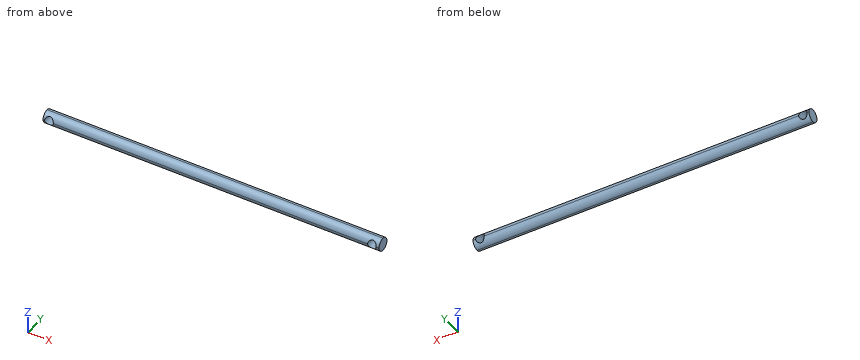
from build123d import *

# Parameters (mm, degrees)
F0_W        = 390
F0_H        = 15
F1_DEPTH    = 15
F2_R        = 5
F3_DEPTH    = 20
F4_T1_DEPTH = 430


# Not quite as in the source:
# - a fillet or chamfer that OpenCascade refuses, or shapes differently, is made with other operations: its cross-section is extruded or revolved along the edge and cut away or added


with BuildPart() as f1:
    # F0 (on Front) → F1 (new body)
    with BuildSketch(Plane.XZ):
        with Locations((-195, 7.5)):
            Rectangle(F0_W, F0_H)
    extrude(amount=F1_DEPTH)

    # F2 (on Front) → F3 (cut)
    with BuildSketch(Plane.XZ):
        with Locations((-383.0693596974, 7.6079843566)):
            Circle(F2_R)
        with Locations((-8.0693596974, 7.6553751715)):
            Circle(F2_R)
    extrude(amount=F3_DEPTH, mode=Mode.SUBTRACT)

    # F4: fillet of radius 8 on 4 edges, made by hand

    # F4_s2 → F4_t1 (cut)
    with BuildSketch(Plane.YZ.offset(-410)):
        with BuildLine():
            ThreePointArc((-8, 15), (-2.3431457505, 12.6568542495), (0, 7))
            Line((0, 7), (0, 15))
            Line((0, 15), (-8, 15))
        make_face()
        with BuildLine():
            ThreePointArc((0, 8), (-2.3431457505, 2.3431457505), (-8, 0))
            Line((-8, 0), (0, 0))
            Line((0, 0), (0, 8))
        make_face()
        with BuildLine():
            ThreePointArc((-7, 15), (-12.6568542495, 12.6568542495), (-15, 7))
            Line((-15, 7), (-15, 15))
            Line((-15, 15), (-7, 15))
        make_face()
        with BuildLine():
            ThreePointArc((-15, 8), (-12.6568542495, 2.3431457505), (-7, 0))
            Line((-7, 0), (-15, 0))
            Line((-15, 0), (-15, 8))
        make_face()
    extrude(amount=F4_T1_DEPTH, mode=Mode.SUBTRACT)


solid = f1.part
Check sheet for the modelled part. Datum: model origin and axes. Units: mm. Round coordinates to 2 decimals unless told otherwise and drop trailing zeros. Loops run counter-clockwise (first coordinate to the right, second up) from the corner with the lowest first, then second, coordinate; pieces in that order, holes last. Notation, with made-up numbers: (51.5, 17) - (91.5, 17) arc R10 ccw to (91.5, 23) - close; hole circle Ø7 at (-35.5, -4). An arc over 180 degrees is marked (long way). Answer as CSV lines item,"result". Start each with the question number.
Item 1: Scan lines: line 1 (X direction, y = -13.25, z = 7.75); line 2 (X direction, y = -13.25, z = 5.25); line 3 (Y direction, x = -104, z = 7.75). Record each from-to range of solid material in increasing order. Write a range as [from, to].
Item 2: Section check B-B (x = -92). Record the boundary of the cut face in (y, z).
Item 3: Depth check by flat-ended pin: P1, Ø5, axis at x = -252, y = -2.5, coming from the +Z side; P2, Ø1.5, axis at x = -47.5, y = -12.5, coming from the +Z side; P3, Ø5, axis at x = -276, z = 4.5, coming from the -Y side; P4, Ø3, axis at y = -3, z = 4, coming from the +X side. Enter the tip coordinate at first touch or a pass-through.
Item 4: Section check A-A (y = -11.25). Record the boundary of the cut face in (x, z).
Report:
1,line 1,"x = [-390, -388.07], [-378.07, -13.07], [-3.07, 0]"
1,line 2,"x = [-390, -387.48], [-378.66, -12.45], [-3.69, 0]"
1,line 3,"y = [-14.96, -0.04]"
2,outline,"(-14.98, 7.5) arc R8 ccw to (-7.5, 0.02) arc R8 ccw to (-0.02, 7.5) arc R8 ccw to (-7.5, 14.98) arc R8 ccw to start"
3,P1,"stops at z = 14.42"
3,P2,"stops at z = 13.44"
3,P3,"stops at y = -14.94"
3,P4,"stops at x = 0"
4,outline,"(-390, 1.22) - (0, 1.22) - (0, 13.78) - (-390, 13.78) - close; hole circle Ø10 at (-383.07, 7.61); hole circle Ø10 at (-8.07, 7.66)"
